from build123d import *

# Parameters (mm, degrees)
BOSS_EXTRUDE1_DEPTH   = 6.35
CUT_EXTRUDE1_DEPTH    = 306.7995770016471
SKETCH3_R             = 7.500000000000012
CUT_EXTRUDE2_DEPTH    = 306.7242323837137
M6X1_0_TAPPED_HOLE1_D = 5
CUT_EXTRUDE4_DEPTH    = 10
SKETCH8_R             = 1.9999999999998708
SKETCH8_R_2           = 2.0000000000000036
SKETCH8_R_3           = 2.00000000000001
SKETCH8_R_4           = 1.9999999999999967
SKETCH8_R_5           = 2.0000000000000275
SKETCH8_R_6           = 1.9999999999999787
CUT_EXTRUDE5_DEPTH    = 10
SKETCH9_R             = 6.000000000000016
CUT_EXTRUDE6_DEPTH    = 10


with BuildPart() as part:
    # Sketch1 → Boss-Extrude1 (new body)
    with BuildSketch(Plane(origin=(0, 0, 0), x_dir=(1, 0, 0), z_dir=(0, 1, 0))):
        with BuildLine():
            Line((6.787858850574763, 64.64460512853856), (264.94156719392146, 37.537765655966744))
            ThreePointArc((264.94156719392146, 37.537765655966744), (298.7441359999997, 0), (264.94156719392146, -37.53776565596673))
            Line((264.94156719392146, -37.53776565596673), (6.787858850574784, -64.64460512853856))
            ThreePointArc((6.787858850574784, -64.64460512853856), (-65, 7.96e-15), (6.787858850574763, 64.64460512853856))
        make_face()
    extrude(amount=BOSS_EXTRUDE1_DEPTH)

    # Sketch2 → Cut-Extrude1 (cut, through all)
    with BuildSketch(Plane(origin=(0, 6.35, 0), x_dir=(1, 0, 0), z_dir=(0, 1, 0))):
        with BuildLine():
            Line((130.0180329989465, 36.62263756219651), (39.67304235209024, 46.10910659001378))
            ThreePointArc((39.67304235209024, 46.10910659001378), (33.61309581948125, 42.68718960147752), (34.86292032668156, 35.84099309862177))
            ThreePointArc((34.86292032668156, 35.84099309862177), (42.769548288999374, 25.89914552943688), (47.915742374995496, 14.285714285714283))
            ThreePointArc((47.915742374995496, 14.285714285714283), (50.07994563199178, 11.189297645576358), (53.665631459994955, 9.999999999999998))
            Line((53.665631459994955, 9.999999999999998), (137.8527855139708, 10.000000000000002))
            ThreePointArc((137.8527855139708, 10.000000000000002), (143.04893793667748, 13.000000000000009), (143.04893793667742, 19.000000000000078))
            Line((143.04893793667742, 19.000000000000078), (134.58761383544618, 33.65544324263917))
            ThreePointArc((134.58761383544618, 33.65544324263917), (132.65904297308322, 35.68763071395833), (130.0180329989465, 36.62263756219651))
        make_face()
        with BuildLine():
            Line((170.26578942302294, 10), (237.1206081654813, 10.000000000000002))
            ThreePointArc((237.1206081654813, 10.000000000000002), (239.94559756005083, 10.706661269050542), (242.10515009108008, 12.660188359810123))
            ThreePointArc((242.10515009108008, 12.660188359810123), (243.00987705511346, 13.915861411150573), (243.9979040786778, 15.107099545201987))
            ThreePointArc((243.9979040786778, 15.107099545201987), (245.10693815146783, 21.261347723744738), (240.1392503071075, 25.05961110306701))
            Line((240.1392503071075, 25.05961110306701), (166.9704585881833, 32.74253266268689))
            ThreePointArc((166.9704585881833, 32.74253266268689), (161.61563702112477, 30.46906980583447), (160.70573127726095, 24.723217483175404))
            Line((160.70573127726095, 24.723217483175404), (164.6276336983075, 13.94787914004592))
            ThreePointArc((164.6276336983075, 13.94787914004592), (166.82433080491668, 11.085087734266024), (170.26578942302294, 10))
        make_face()
        with BuildLine():
            Line((170.26578942302294, -10), (237.1206081654813, -10.000000000000002))
            ThreePointArc((237.1206081654813, -10.000000000000002), (239.94559756005083, -10.706661269050542), (242.10515009108008, -12.660188359810123))
            ThreePointArc((242.10515009108008, -12.660188359810123), (243.00987705511346, -13.915861411150573), (243.9979040786778, -15.107099545201987))
            ThreePointArc((243.9979040786778, -15.107099545201987), (245.10693815146783, -21.261347723744738), (240.1392503071075, -25.05961110306701))
            Line((240.1392503071075, -25.05961110306701), (166.9704585881833, -32.74253266268689))
            ThreePointArc((166.9704585881833, -32.74253266268689), (161.61563702112477, -30.46906980583447), (160.70573127726095, -24.723217483175404))
            Line((160.70573127726095, -24.723217483175404), (164.6276336983075, -13.94787914004592))
            ThreePointArc((164.6276336983075, -13.94787914004592), (166.82433080491668, -11.085087734266024), (170.26578942302294, -10))
        make_face()
        with BuildLine():
            Line((130.01803299894652, -36.622637562196495), (39.67304235209024, -46.10910659001378))
            ThreePointArc((39.67304235209024, -46.10910659001378), (33.61309581948125, -42.68718960147752), (34.86292032668156, -35.84099309862177))
            ThreePointArc((34.86292032668156, -35.84099309862177), (42.769548288999374, -25.89914552943688), (47.915742374995496, -14.285714285714283))
            ThreePointArc((47.915742374995496, -14.285714285714283), (50.07994563199178, -11.189297645576358), (53.665631459994955, -9.999999999999998))
            Line((53.665631459994955, -9.999999999999998), (137.8527855139708, -10))
            ThreePointArc((137.8527855139708, -10), (143.04893793667745, -13.000000000000027), (143.0489379366774, -19.000000000000057))
            Line((143.0489379366774, -19.000000000000057), (134.58761383544623, -33.65544324263918))
            ThreePointArc((134.58761383544623, -33.65544324263918), (132.65904297308327, -35.687630713958356), (130.01803299894652, -36.622637562196495))
        make_face()
        with BuildLine():
            ThreePointArc((6.787858850574784, -64.64460512853856), (-36.35930093139005, 2.251e-14), (6.787858850574836, 64.64460512853859))
            ThreePointArc((6.787858850574836, 64.64460512853859), (-65.00000000000003, 3.683e-14), (6.787858850574784, -64.64460512853856))
        make_face()
    extrude(amount=-CUT_EXTRUDE1_DEPTH, mode=Mode.SUBTRACT)

    # Sketch3 → Cut-Extrude2 (cut, through all)
    with BuildSketch(Plane(origin=(0, 6.35, 0), x_dir=(1, 0, 0), z_dir=(0, 1, 0))):
        with Locations(Location((261, 0, 0), (0, 0, 270))):
            Circle(SKETCH3_R)
        with BuildLine():
            Line((3.0000000000000004, 5.65685424949238), (3.0000000000000004, -5.65685424949238))
            ThreePointArc((3.0000000000000004, -5.65685424949238), (2.8164965809277267, -6.234204518682005), (2.333333333333334, -6.599663291074442))
            ThreePointArc((2.333333333333334, -6.599663291074442), (-6.999999999999999, 8.6e-16), (2.333333333333334, 6.599663291074442))
            ThreePointArc((2.333333333333334, 6.599663291074442), (2.8164965809277267, 6.234204518682005), (3.0000000000000004, 5.65685424949238))
        make_face()
    extrude(amount=-CUT_EXTRUDE2_DEPTH, mode=Mode.SUBTRACT)

    # M6x1.0 Tapped Hole1 (through all)
    with Locations(Plane(origin=(0, 6.35, 0), x_dir=(1, 0, 0), z_dir=(0, 1, 0))):
        with Locations((0, 20), (20, 0), (0, -20), (-20, 0), (276, 0), (246.00004616, 0.037212923), (246, 0), (260.510261233, 14.992003066), (260.510261233, -14.992003066)):
            Hole(M6X1_0_TAPPED_HOLE1_D / 2)

    # Sketch7 → Cut-Extrude4 (cut)
    with BuildSketch(Plane(origin=(0, 6.35, 0), x_dir=(1, 0, 0), z_dir=(0, 1, 0))):
        with BuildLine():
            Line((261.0000005017777, -7.5), (256, -7.5))
            ThreePointArc((256, -7.5), (251.2288142968451, -5.786690503734399), (248.63750000000002, -1.42954319626934))
            ThreePointArc((248.63750000000002, -1.42954319626934), (247.53482452006037, -2.577656628145443), (246.00000083547474, -3.0000000000000013))
            Line((246.00000083547474, -3.0000000000000013), (240, -3.000000000000001))
            ThreePointArc((240, -3.000000000000001), (236.99999999999991, -4.1773736761e-07), (239.99999916452526, 3.0000000000000004))
            Line((239.99999916452526, 3.0000000000000004), (246, 3))
            ThreePointArc((246, 3), (247.53482416113246, 2.577656841863176), (248.63750000000002, 1.42954319626934))
            ThreePointArc((248.63750000000002, 1.42954319626934), (251.2288141032696, 5.786690344129463), (255.99999949822234, 7.5))
            Line((255.99999949822234, 7.5), (261, 7.5))
            ThreePointArc((261, 7.5), (265.39806452485095, 6.07511550797577), (268.125, 2.341874249399391))
            ThreePointArc((268.125, 2.341874249399391), (269.0064263359464, 2.830690971140985), (270, 3))
            Line((270, 3), (276, 3))
            ThreePointArc((276, 3), (279, 0), (276, -3))
            Line((276, -3), (270, -3))
            ThreePointArc((270, -3), (269.0064263359464, -2.8306909711409793), (268.125, -2.341874249399391))
            ThreePointArc((268.125, -2.341874249399391), (265.39806472807476, -6.075115360852396), (261.0000005017777, -7.5))
        make_face()
        with BuildLine():
            Line((260.51026123316717, -17.992003066310435), (254.51026123316717, -17.99200306631043))
            ThreePointArc((254.51026123316717, -17.99200306631043), (251.51026123316717, -14.992003066310435), (254.51026123316717, -11.992003066310438))
            Line((254.51026123316717, -11.992003066310438), (260.51026123316717, -11.992003066310433))
            ThreePointArc((260.51026123316717, -11.992003066310433), (263.51026123316717, -14.992003066310435), (260.51026123316717, -17.992003066310435))
        make_face()
        with BuildLine():
            Line((261, 12.000000000000014), (255, 12.00000000000001))
            ThreePointArc((255, 12.00000000000001), (252, 15.000000000000012), (255, 18.000000000000014))
            Line((255, 18.000000000000014), (261, 18.000000000000014))
            ThreePointArc((261, 18.000000000000014), (264, 15.000000000000014), (261, 12.000000000000014))
        make_face()
    extrude(amount=-CUT_EXTRUDE4_DEPTH, mode=Mode.SUBTRACT)

    # Sketch8 → Cut-Extrude5 (cut)
    with BuildSketch(Plane(origin=(0, 6.35, 0), x_dir=(1, 0, 0), z_dir=(0, 1, 0))):
        with Locations(Location((35.6282598801996, -54.07505226292096, 0), (0, 0, 270))):
            Circle(SKETCH8_R)
        with Locations(Location((60.49156954502199, -51.46433732039219, 0), (0, 0, 270))):
            Circle(SKETCH8_R_2)
        with Locations(Location((85.35487920984451, -48.853622377863424, 0), (0, 0, 270))):
            Circle(SKETCH8_R_3)
        with Locations(Location((110.21818887466702, -46.24290743533465, 0), (0, 0, 270))):
            Circle(SKETCH8_R_4)
        with Locations(Location((135.08149853948953, -43.63219249280589, 0), (0, 0, 270))):
            Circle(SKETCH8_R_5)
        with Locations(Location((159.9448082043121, -41.02147755027711, 0), (0, 0, 270))):
            Circle(SKETCH8_R_4)
        with Locations(Location((184.8081178691346, -38.41076260774834, 0), (0, 0, 270))):
            Circle(SKETCH8_R_4)
        with Locations(Location((209.67142753395711, -35.80004766521956, 0), (0, 0, 270))):
            Circle(SKETCH8_R_4)
        with Locations(Location((234.53473719877965, -33.1893327226908, 0), (0, 0, 270))):
            Circle(SKETCH8_R_4)
        with Locations(Location((234.53473719877965, 33.1893327226908, 0), (0, 0, 270))):
            Circle(SKETCH8_R_4)
        with Locations(Location((209.67142753395711, 35.80004766521956, 0), (0, 0, 270))):
            Circle(SKETCH8_R_4)
        with Locations(Location((184.8081178691346, 38.41076260774834, 0), (0, 0, 270))):
            Circle(SKETCH8_R_4)
        with Locations(Location((159.9448082043121, 41.02147755027711, 0), (0, 0, 270))):
            Circle(SKETCH8_R_4)
        with Locations(Location((135.08149853948953, 43.63219249280589, 0), (0, 0, 270))):
            Circle(SKETCH8_R_5)
        with Locations(Location((110.21818887466702, 46.24290743533465, 0), (0, 0, 270))):
            Circle(SKETCH8_R_4)
        with Locations(Location((85.35487920984451, 48.853622377863424, 0), (0, 0, 270))):
            Circle(SKETCH8_R_3)
        with Locations(Location((60.49156954502199, 51.46433732039219, 0), (0, 0, 270))):
            Circle(SKETCH8_R_2)
        with Locations(Location((35.628259880199494, 54.07505226292097, 0), (0, 0, 270))):
            Circle(SKETCH8_R_6)
    extrude(amount=-CUT_EXTRUDE5_DEPTH, mode=Mode.SUBTRACT)

    # Sketch9 → Cut-Extrude6 (cut)
    with BuildSketch(Plane(origin=(0, 6.35, 0), x_dir=(1, 0, 0), z_dir=(0, 1, 0))):
        with Locations(Location((155, 0, 0), (0, 0, 270))):
            Circle(SKETCH9_R)
    extrude(amount=-CUT_EXTRUDE6_DEPTH, mode=Mode.SUBTRACT)


solid = part.part
Source: CAD feature listing. Evaluate the final solid. Frame: model axes, mm. Give positions to 0.01 mm unless a question says otherwise; leave off trailing zeros. Write each loop counter-clockwise with the first axis right and the second up, starting at its lowest first coordinate (ties: lowest second). Pieces come first, ordered by that corner, then holes. Notation, with made-up numbers: (66.25, 35) -> (89.25, 35) arc R9 ccw to (89.25, 39) -> close; hole circle Ø4 at (18, 51.25). An arc over 180 degrees is marked (long way). Return JSON: item names as keys, results as strings. Group by question number.
1. Material intervals for line 1 (X direction, y = 5, z = 15); line 2 (Z direction, x = 36, y = 4.5); line 3 (X direction, y = 6.25, z = 0.5), sorted ascending. Write a range as from..to.
2. Section A-A, the plane x = 155. Output: boundary loops of the cut face in (y, z).
3. Section B-B, the plane y = 2. Count the separate pieces of the cut face and the enclosed holes in it, then the cut area to 3 significant figures.
4. Pin query (flat end, axial travel): pin 1 Ø1.9 at (x, y) = (190.5, 2) entering from +Z; pin 2 Ø3 at (x, z) = (234.53, -33.19) entering from -Y; pin 3 Ø2 at (x, y) = (253, 5) entering from -Z; pin 4 Ø1.5 at (x, y) = (258.5, 4) entering from +Z. Return the tip coordinate at first contact, or that it passes through.
5. Mould query, pull axis Z, two halves, no side actions, for faces 1 (the face through (137.7, 3.1, 50.9)), 2 (the face through (3, 3, 0)). Classes: +Z half, -Z half, draft (parallel to the pull), parting line (faces both ways), or undercut.
Determined:
{
 "1": {"line 1": "x = -34.73..47.7, 143.77..164.24, 243.9..251.51, 263.51..295.64", "line 2": "z = -61.58..-56.04, -52.11..-45.31, -34.7..34.7, 45.31..52.11, 56.04..61.58", "line 3": "x = -36.36..-22.45, -17.55..-6.98, 3..17.55, 22.45..149.02, 160.98..237.04, 278.96..298.74"},
 "2": {"outline": "(0, -49.08) -> (6.35, -49.08) -> (6.35, -6) -> (0, -6) -> close; (0, 6) -> (6.35, 6) -> (6.35, 49.08) -> (0, 49.08) -> close"},
 "3": {"separate pieces": "1", "enclosed holes": "31", "area": "22,200 mm2"},
 "4": {"pin 1": "stops at z = 45.45", "pin 2": "passes through", "pin 3": "stops at z = -38.9", "pin 4": "stops at z = 38.29"},
 "5": {"face 1": "+Z half", "face 2": "undercut"}
}
